from build123d import *

# Parameters (mm, degrees)
SKETCH1_R           = 2
BOSS_EXTRUDE1_DEPTH = 3
CHAMFER1_SIZE       = 0.5


with BuildPart() as part:
    # Sketch1 → Boss-Extrude1 (new body)
    with BuildSketch(Plane.XY):
        Polygon((4.330127019, 0), (2.165063509, 3.75), (-2.165063509, 3.75), (-4.330127019, 0), (-2.165063509, -3.75), (2.165063509, -3.75), align=None)
        Circle(SKETCH1_R, mode=Mode.SUBTRACT)
    extrude(amount=BOSS_EXTRUDE1_DEPTH)

    # Sketch2 → Cut-Revolve1 (revolve, cut)
    with BuildSketch(Plane(origin=(0, 0, 0), x_dir=(1, 0, 0), z_dir=(0, 1, 0)), mode=Mode.PRIVATE) as cut_revolve1_sk:
        with BuildLine():
            Line((-4.330127019, -1.952562419), (-6.415307532, -1.952562419))
            ThreePointArc((-6.415307532, -1.952562419), (-3.99218262, -5.388056111), (0, -6.70586838))
            Line((0, -6.70586838), (0, -4.75))
            ThreePointArc((0, -4.75), (-2.577579146, -3.989810239), (-4.330127019, -1.952562419))
        make_face()
    cut_revolve1 = revolve(cut_revolve1_sk.sketch.rotate(Axis((0, 0, 1.952562419), (0, 0, 1)), 180), axis=Axis((0, 0, 1.952562419), (0, 0, 1)), mode=Mode.SUBTRACT)

    # Mirror1: Cut-Revolve1 across plane
    add(cut_revolve1.mirror(Plane(origin=(0, 0, 1.5), x_dir=(1, 0, 0), z_dir=(0, 0, -1))), mode=Mode.SUBTRACT)

    # Chamfer1
    chamfer1_edges = [part.edges().sort_by_distance(p)[0] for p in [
        (-2, 0, 0),
        (-2, 0, 3),
    ]]
    chamfer(chamfer1_edges, length=CHAMFER1_SIZE)


solid = part.part
Geometry check sheet. Reference: the model listing, model coordinates, mm. Give positions to 0.01 mm unless a question says otherwise; leave off trailing zeros. Order: outer loops, then holes, each group sorted by start corner. A loop starts at its lowest first (then second) coordinate and runs counter-clockwise, first axis right, second up. Notation, with made-up numbers: (88.5, 10) - (137.5, 10) arc R20 ccw to (137.5, 46) - close; hole circle Ø6 at (-28, -33.75). An arc over 180 degrees is marked (long way). Answer as a JSON object with one key per item and string values.
(1) Cross-section at D-D (z = 0.3). Record the cut outline in (x, y).
Report:
{"outline": "(-3.8, -0.92) - (-2.7, -2.83) arc R3.91 ccw to (-1.1, -3.75) - (1.1, -3.75) arc R3.91 ccw to (2.7, -2.83) - (3.8, -0.92) arc R3.91 ccw to (3.8, 0.92) - (2.7, 2.83) arc R3.91 ccw to (1.1, 3.75) - (-1.1, 3.75) arc R3.91 ccw to (-2.7, 2.83) - (-3.8, 0.92) arc R3.91 ccw to start; hole circle Ø4.4 at (0, 0)"}
(2) Cross-section at C-C (x = 3.5). Record the cut outline in (y, z), then the cut area to 3 significant figures.
Report:
{"outline": "(-1.44, 0.13) arc R3.21 ccw to (-1.15, 0) - (1.15, 0) arc R3.21 ccw to (1.44, 0.13) - (1.44, 2.87) arc R3.21 ccw to (1.15, 3) - (-1.15, 3) arc R3.21 ccw to (-1.44, 2.87) - close", "area": "8.56 mm^2"}
(3) Depth check by flat-ended pin: pin 1 Ø1 at (x, y) = (-3, -2) entering from -Z. Enter the tip coordinate at first touch or a pass-through.
Report:
{"pin 1": "z = 0"}
(4) Draft check along Y on faces 1 (the cylindrical face through (0, -2, 1)), 2 (the flat face through (0, -3.75, 1)), 3 (the flat face through (3.26, 1.85, 1.48)). Enter one of: released by +Y, released by -Y, zero draft, split by the parting line, or undercut.
Report:
{"face 1": "undercut", "face 2": "released by -Y", "face 3": "released by +Y"}
(5) Material ranges on line 1 (Y direction, x = 0, z = 1.8); line 2 (Y direction, x = 1.5, z = 2.35); line 3 (X direction, y = 1.25, z = 2.35), recorded low to high.
Report:
{"line 1": "-3.75 to -2, 2 to 3.75", "line 2": "-3.75 to -1.32, 1.32 to 3.75", "line 3": "-3.61 to -1.56, 1.56 to 3.61"}
(6) Cross-section at A-A (x = 0). Record the cut outline in (y, z).
Report:
{"outline": "(-3.75, 0.08) arc R4.75 ccw to (-3.68, 0) - (-2.5, 0) - (-2, 0.5) - (-2, 2.5) - (-2.5, 3) - (-3.68, 3) arc R4.75 ccw to (-3.75, 2.92) - close; (2, 0.5) - (2.5, 0) - (3.68, 0) arc R4.75 ccw to (3.75, 0.08) - (3.75, 2.92) arc R4.75 ccw to (3.68, 3) - (2.5, 3) - (2, 2.5) - close"}
(7) Cross-section at B-B (z = 1.45). Record the cut outline in (x, y), then the cut area to 3 significant figures.
Report:
{"outline": "(-4.33, 0) - (-2.17, -3.75) - (2.17, -3.75) - (4.33, 0) - (2.17, 3.75) - (-2.17, 3.75) - close; hole circle Ø4 at (0, 0)", "area": "36.1 mm^2"}
